The listing builds one solid part. Answer for the finished solid, in the listing's coordinates (mm). A direction names the side the tool comes from. Round coordinates to 2 decimals unless told otherwise and drop trailing zeros. Loops run counter-clockwise (first coordinate to the right, second up) from the corner with the lowest first, then second, coordinate; pieces in that order, holes last. Notation, with made-up numbers: (66.5, 39.5) -> (119.5, 39.5) arc R25 ccw to (119.5, 55.5) -> close; hole circle Ø10 at (-0.75, -4.5). An arc over 180 degrees is marked (long way). Use a Markdown table: item, result. Add a question column.
Q1. Section C-C on z = -7.5 is taken. Give the vertices of the cut face in (x, y).
Q2. For a pull along X with two mould halves and no side action, classify faces 4 (the cylindrical face through (15.69, 0.04, 1.97)), 5 (the flat face through (-10.319, 0, 32)), 6 (the cylindrical face through (-11.233, -0.067, -2.494)) as released by +X, released by -X, zero draft, split by the parting line, or undercut.
Q3. Section B-B on x = 0 is taken. Give the vertices of the cut face in (y, z), then the cut area to 3 significant figures.
Q4. Given pin 1 Ø10 at (x, z) = (12.5, 17.5) entering from +Y; pin 2 Ø3 at (y, z) = (-0.5, 29.5) entering from -X; pin 3 Ø1 at (x, z) = (27, 19) entering from -Y; pin 4 Ø18.5 at (x, z) = (0, 0) entering from -Y, each flat-ended and moving along its own axis, determine where each tip first touches the part or whether it passes through.
Q5. Section D-D on z = 28 is taken. Give the vertices of the cut face in (x, y), then the cut area to 3 significant figures.
Q6. Section A-A on y = 0.5 is taken. Give the vertices of the cut face in (x, z) (1 decimal).
Q7. Consider line 1 (X direction, y = 0.75, z = 36); line 2 (X direction, y = -0.5, z = 23.5); line 3 (Z direction, x = 0.5, y = -0.75). Determine where each line is inside the solid, lowest interval first.
Q8. Which of the six approach directions +Z, -Z, +X, -X, +Y, -Y give full straight-line access (tool end or side, diameter ignored) to faces 1 (the cylindrical face through (-9.87, 0.04, 48.91)), 2 (the flat face through (-5.556, 0, 32)), 3 (the flat face through (10.319, 0, 41))?
from build123d import *

# Parameters (mm, degrees)
BOSS_EXTRUDE1_DEPTH      = 4.7625
BOSS_EXTRUDE1_DEPTH_BACK = 4.7625
SKETCH1_R                = 14.6812
SKETCH1_R_2              = 11.5062
BOSS_EXTRUDE2_DEPTH      = 2.9972
BOSS_EXTRUDE2_DEPTH_BACK = 2.9972
FILLET1_R                = 16.002
FILLET2_R                = 1.5875


with BuildPart() as part:
    # Sketch1 → Boss-Extrude1 (new, two sides: drawn at the far end of the back side and taken through both)
    with BuildSketch(Plane(origin=(0, 0, 0), x_dir=(1, 0, 0), z_dir=(0, 1, 0)).offset(-BOSS_EXTRUDE1_DEPTH_BACK)):
        with Locations(Location((0, 0, 0), (0, 0, 270))):
            Circle(SKETCH1_R)
        with Locations(Location((0, 0, 0), (0, 0, 270))):
            Circle(SKETCH1_R_2, mode=Mode.SUBTRACT)
    extrude(amount=BOSS_EXTRUDE1_DEPTH + BOSS_EXTRUDE1_DEPTH_BACK)

    # Sketch1<4> → Boss-Extrude2 (add, two sides: drawn at the far end of the back side and taken through both)
    with BuildSketch(Plane(origin=(0, 0, 0), x_dir=(1, 0, 0), z_dir=(0, 1, 0)).offset(-BOSS_EXTRUDE2_DEPTH_BACK)):
        with BuildLine():
            Line((-10.31875, -10.443228997), (-10.31875, -49.3903))
            Line((-10.31875, -49.3903), (10.31875, -49.3903))
            Line((10.31875, -49.3903), (10.31875, -28.986981317))
            Line((10.31875, -28.986981317), (23.211292264, -44.800828643))
            Line((23.211292264, -44.800828643), (39.206644749, -31.760310817))
            Line((39.206644749, -31.760310817), (14.596591512, -1.573896333))
            ThreePointArc((14.596591512, -1.573896333), (4.923540137, -13.830993672), (-10.31875, -10.443228997))
        make_face()
        with BuildLine():
            Line((-5.55625, -39.07155), (-5.55625, -25.48255))
            ThreePointArc((-5.55625, -25.48255), (0, -19.9263), (5.55625, -25.48255))
            Line((5.55625, -25.48255), (5.55625, -39.07155))
            ThreePointArc((5.55625, -39.07155), (0, -44.6278), (-5.55625, -39.07155))
        make_face(mode=Mode.SUBTRACT)
        with BuildLine():
            Line((20.38226854, -33.793802133), (11.795589111, -23.261477728))
            ThreePointArc((11.795589111, -23.261477728), (12.591121519, -15.444128029), (20.408471218, -16.239660438))
            Line((20.408471218, -16.239660438), (28.995150647, -26.771984843))
            ThreePointArc((28.995150647, -26.771984843), (28.199618239, -34.589334541), (20.38226854, -33.793802133))
        make_face(mode=Mode.SUBTRACT)
    extrude(amount=BOSS_EXTRUDE2_DEPTH + BOSS_EXTRUDE2_DEPTH_BACK)

    # Fillet1
    fillet1_edges = [part.edges().sort_by_distance(p)[0] for p in [
        (-10.31875, 0, 10.443228997),
        (14.596591512, 0, 1.573896333),
    ]]
    fillet(fillet1_edges, radius=FILLET1_R)

    # Fillet2
    fillet2_edges = [part.edges().sort_by_distance(p)[0] for p in [
        (39.206644749, 0, 31.760310817),
        (23.211292264, 0, 44.800828643),
        (10.31875, 0, 28.986981317),
        (10.31875, 0, 49.3903),
        (-10.31875, 0, 49.3903),
    ]]
    fillet(fillet2_edges, radius=FILLET2_R)


solid = part.part
Checked values:
| question | item | result |
|---|---|---|
| 1 | outline | (-12.62, -4.76) -> (-8.73, -4.76) -> (-8.73, 4.76) -> (-12.62, 4.76) -> close; (8.73, -4.76) -> (12.62, -4.76) -> (12.62, 4.76) -> (8.73, 4.76) -> close |
| 2 | face 4 | released by +X |
| 2 | face 5 | released by -X |
| 2 | face 6 | undercut |
| 3 | outline | (-4.76, -14.68) -> (4.76, -14.68) -> (4.76, -11.51) -> (-4.76, -11.51) -> close; (-4.76, 11.51) -> (4.76, 11.51) -> (4.76, 14.68) -> (3, 14.68) -> (3, 19.93) -> (-3, 19.93) -> (-3, 14.68) -> (-4.76, 14.68) -> close; (-3, 44.63) -> (3, 44.63) -> (3, 49.39) -> (-3, 49.39) -> close |
| 3 | area | 120 mm2 |
| 4 | pin 1 | stops at y = 3 |
| 4 | pin 2 | stops at x = -10.32 |
| 4 | pin 3 | stops at y = -3 |
| 4 | pin 4 | passes through |
| 5 | outline | (-10.32, -3) -> (-5.56, -3) -> (-5.56, 3) -> (-10.32, 3) -> close; (5.56, -3) -> (15.66, -3) -> (15.66, 3) -> (5.56, 3) -> close; (29.75, -3) -> (36.14, -3) -> (36.14, 3) -> (29.75, 3) -> close |
| 5 | area | 127 mm2 |
| 6 | outline | (-12.6, 7.5) arc R14.7 ccw (long way) to (14.5, -2.1) arc R16 cw to (18, 5.7) -> (38.2, 30.5) arc R1.6 ccw to (38, 32.8) -> (24.4, 43.8) arc R1.6 ccw to (22.2, 43.6) -> (13.1, 32.4) arc R1.6 cw to (10.3, 33.4) -> (10.3, 47.8) arc R1.6 ccw to (8.7, 49.4) -> (-8.7, 49.4) arc R1.6 ccw to (-10.3, 47.8) -> (-10.3, 15.8) arc R16 cw to start; hole circle Ø23 at (0, 0); hole (-5.6, 25.5) arc R5.6 ccw to (5.6, 25.5) -> (5.6, 39.1) arc R5.6 ccw to (-5.6, 39.1) -> close; hole (11.8, 23.3) arc R5.6 ccw to (20.4, 16.2) -> (29, 26.8) arc R5.6 ccw to (20.4, 33.8) -> close |
| 7 | line 1 | x = -10.32 to -5.56, 5.56 to 10.32, 16.04 to 34.01 |
| 7 | line 2 | x = -10.32 to -5.19, 5.19 to 11.99, 26.33 to 32.47 |
| 7 | line 3 | z = -14.67 to -11.5, 11.5 to 19.95, 44.61 to 49.39 |
| 8 | face 1 | +Z, -X, +Y, -Y |
| 8 | face 2 | +Y, -Y |
| 8 | face 3 | +Z, +Y, -Y |
